Here's how the part is built. I have some questions about the finished solid (model axes, mm). Face numbers are marked on the shaded views. A direction names the side the tool comes from. Round coordinates to 2 decimals unless told otherwise and drop trailing zeros. Order: outer loops, then holes, each group sorted by start corner. A loop starts at its lowest first (then second) coordinate and runs counter-clockwise, first axis right, second up.
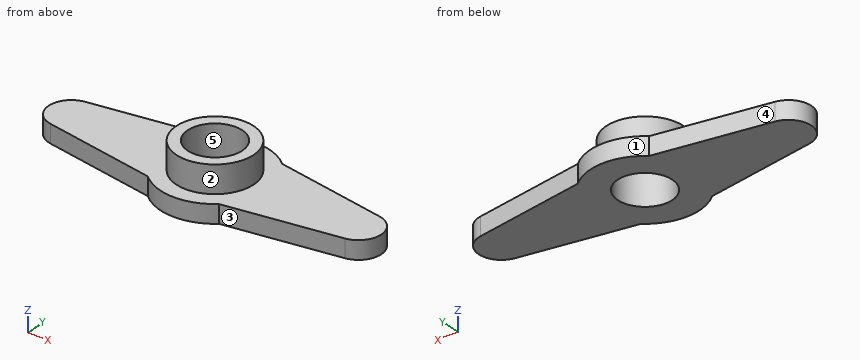
```python
from build123d import *

# Parameters (mm, degrees)
BOSS_EXTRUDE1_DEPTH = 2
SKETCH2_R           = 4.25
BOSS_EXTRUDE2_DEPTH = 3
CUT_EXTRUDE1_REACH  = 22.081
SKETCH3_R           = 3


with BuildPart() as part:
    # Sketch1 → Boss-Extrude1 (new body)
    with BuildSketch(Plane.XY):
        with BuildLine():
            Line((-3.963767369, 4.504281102), (-16.404004536, 2.467140112))
            ThreePointArc((-16.404004536, 2.467140112), (-18.5, -1e-09), (-16.404004536, -2.467140113))
            Line((-16.404004536, -2.467140113), (-3.963767369, -4.504281102))
            ThreePointArc((-3.963767369, -4.504281102), (0, -6), (3.963767369, -4.504281102))
            Line((3.963767369, -4.504281102), (16.404004536, -2.467140112))
            ThreePointArc((16.404004536, -2.467140112), (18.5, 0), (16.404004536, 2.467140113))
            Line((16.404004536, 2.467140113), (3.963767369, 4.504281102))
            ThreePointArc((3.963767369, 4.504281102), (0, 6), (-3.963767369, 4.504281102))
        make_face()
    extrude(amount=BOSS_EXTRUDE1_DEPTH)

    # Sketch2 → Boss-Extrude2 (add)
    with BuildSketch(Plane.XY.offset(2)):
        Circle(SKETCH2_R)
    extrude(amount=BOSS_EXTRUDE2_DEPTH)

    # Sketch3 → Cut-Extrude1 (cut, up to next)
    with BuildSketch(Plane(origin=(0, 0, 0), x_dir=(-1, 0, 0), z_dir=(0, 0, -1)), mode=Mode.PRIVATE) as cut_extrude1_sk1:
        Circle(SKETCH3_R)
    cut_extrude1_tool1 = extrude(cut_extrude1_sk1.sketch, amount=-CUT_EXTRUDE1_REACH, mode=Mode.PRIVATE) & part.part
    add(cut_extrude1_tool1.solids().sort_by_distance((0, 0, 0))[0], mode=Mode.SUBTRACT)


solid = part.part
```
1. If we section it at A-A, the plane y = 0: Write out the boundary of the cut face in (x, z), and give its area (3 significant figures).
Evaluation:
outline: (-18.5, 0) - (-3, 0) - (-3, 5) - (-4.25, 5) - (-4.25, 2) - (-18.5, 2) - close; (3, 0) - (18.5, 0) - (18.5, 2) - (4.25, 2) - (4.25, 5) - (3, 5) - close
area: 69.5 mm2
2. If we section it at C-C, the plane z = 2.35: Write out the boundary of the cut face in (x, y), and give its area (3 significant figures).
Evaluation:
outline: circle Ø8.5 at (0, 0); hole circle Ø6 at (0, 0)
area: 28.5 mm2
3. I'm going to push flat-ended pins straight in: P1, Ø5, axis at x = 9, y = 2.5, coming from the -Z side; P2, Ø5.5, axis at x = 0, y = 0, coming from the +Z side; P3, Ø4, axis at x = 9.5, y = 0, coming from the +Z side. Where does each tip first touch, or does it pass through?
Evaluation:
P1: stops at z = 0
P2: passes through
P3: stops at z = 2
4. If we mould it in two halves opening along X, with no side actions, what happens to the marked faces 3, 4 and 5? For each: released by +X, released by -X, zero draft, split by the parting line, or undercut.
Evaluation:
face 3: released by +X
face 4: released by -X
face 5: undercut
5. If we section it at B-B, the plane x = 0: Write out the boundary of the cut face in (y, z), and give its area (3 significant figures).
Evaluation:
outline: (-6, 0) - (-3, 0) - (-3, 5) - (-4.25, 5) - (-4.25, 2) - (-6, 2) - close; (3, 0) - (6, 0) - (6, 2) - (4.25, 2) - (4.25, 5) - (3, 5) - close
area: 19.5 mm2
6. If we section it at D-D, the plane x = 16: Write out the boundary of the cut face in (y, z), and give its area (3 significant figures).
Evaluation:
outline: (-2.53, 0) - (2.53, 0) - (2.53, 2) - (-2.53, 2) - close
area: 10.1 mm2
7. I need wall thicknesses on probe 1 along Y at (x, z) = (0, 3.05); probe 2 along Y at (x, z) = (0, 1.45); probe 3 along Z at (x, y) = (-8.5, 0.75). Which ranges of each line are inside material? Lowest first, please.
Evaluation:
probe 1: y = -4.25 to -3, 3 to 4.25
probe 2: y = -6 to -3, 3 to 6
probe 3: z = 0 to 2
8. On a 3-axis mill with a long thin cutter (end or side, diameter ignored), from which of +Z, -Z, +X, -X, +Y, -Y can I reach the whole of each face in a straight line? I mean the marked faces 1 and 2. Say none if no direction works.
Evaluation:
face 1: +Z, -Z, +Y
face 2: +Z
